Input: part model. Units: mm. Frame: model coordinates. A direction names the side the tool comes from. Coordinates: 2 decimals unless noted, no trailing zeros. Order: outer loops, then holes, each group sorted by start corner. A loop starts at its lowest first (then second) coordinate and runs counter-clockwise, first axis right, second up. Notation, with made-up numbers: M 37.5,1 L 85.5,1 A10 cw 85.5,6 Z; hole C 17,87 d1. An arc over 180 degrees is marked long. Answer in a Markdown table with one row per item.
from build123d import *

# Parameters (mm, degrees)
SKETCH1_R           = 4.198469776
BOSS_EXTRUDE1_DEPTH = 2


with BuildPart() as part:
    # Sketch1 → Boss-Extrude1 (new body)
    with BuildSketch(Plane(origin=(0, 0, 1287.795194646), x_dir=(-1, 0, 0), z_dir=(0, 0, -1))):
        with BuildLine():
            Line((-628.291713491, 871.098927157), (-628.291713491, 890.298927157))
            ThreePointArc((-628.291713491, 890.298927157), (-630.049072803, 894.541567844), (-634.291713491, 896.298927157))
            Line((-634.291713491, 896.298927157), (-714.691713491, 896.298927157))
            ThreePointArc((-714.691713491, 896.298927157), (-718.934354178, 894.541567844), (-720.691713491, 890.298927157))
            Line((-720.691713491, 890.298927157), (-720.691713491, 871.098927157))
            ThreePointArc((-720.691713491, 871.098927157), (-718.934354178, 866.85628647), (-714.691713491, 865.098927157))
            Line((-714.691713491, 865.098927157), (-634.291713491, 865.098927157))
            ThreePointArc((-634.291713491, 865.098927157), (-630.049072803, 866.85628647), (-628.291713491, 871.098927157))
        make_face()
        with Locations((-707.866713491, 880.098927157)):
            Circle(SKETCH1_R, mode=Mode.SUBTRACT)
        with Locations((-641.116713491, 880.098927157)):
            Circle(SKETCH1_R, mode=Mode.SUBTRACT)
        with BuildLine():
            Line((-682.991714253, 882.493927157), (-685.691713491, 882.493927157))
            Line((-685.691713491, 882.493927157), (-685.691713491, 891.298927157))
            Line((-685.691713491, 891.298927157), (-676.886713491, 891.298927157))
            Line((-676.886713491, 891.298927157), (-676.886713491, 888.59892792))
            ThreePointArc((-676.886713491, 888.59892792), (-677.027302174, 888.259516726), (-677.366713318, 888.11892792))
            Line((-677.366713318, 888.11892792), (-679.535834903, 888.118927139))
            ThreePointArc((-679.535834903, 888.118927139), (-680.090162448, 887.748537098), (-679.960098756, 887.09466307))
            Line((-679.960098756, 887.09466307), (-677.620321725, 884.754886039))
            ThreePointArc((-677.620321725, 884.754886039), (-676.705447884, 884.143586882), (-675.626280608, 883.928927162))
            Line((-675.626280608, 883.928927162), (-673.357146389, 883.928927157))
            ThreePointArc((-673.357146389, 883.928927157), (-672.277979107, 884.143586875), (-671.363105261, 884.754886034))
            Line((-671.363105261, 884.754886034), (-669.023328231, 887.094663064))
            ThreePointArc((-669.023328231, 887.094663064), (-668.893264539, 887.748537091), (-669.447592082, 888.118927133))
            Line((-669.447592082, 888.118927133), (-671.616713665, 888.11892792))
            ThreePointArc((-671.616713665, 888.11892792), (-671.956124807, 888.259516727), (-672.096713491, 888.59892792))
            Line((-672.096713491, 888.59892792), (-672.096713491, 891.298927157))
            Line((-672.096713491, 891.298927157), (-663.291713491, 891.298927157))
            Line((-663.291713491, 891.298927157), (-663.291713491, 882.493927157))
            Line((-663.291713491, 882.493927157), (-665.991712728, 882.493927157))
            ThreePointArc((-665.991712728, 882.493927157), (-666.331123921, 882.634515841), (-666.471712728, 882.973926984))
            Line((-666.471712728, 882.973926984), (-666.471713509, 885.14304857))
            ThreePointArc((-666.471713509, 885.14304857), (-666.84210355, 885.697376115), (-667.495977578, 885.567312423))
            Line((-667.495977578, 885.567312423), (-669.835754609, 883.227535392))
            ThreePointArc((-669.835754609, 883.227535392), (-670.447053766, 882.312661551), (-670.661713486, 881.233494275))
            Line((-670.661713486, 881.233494275), (-670.66171349, 878.964360056))
            ThreePointArc((-670.66171349, 878.964360056), (-670.447053773, 877.885192774), (-669.835754613, 876.970318927))
            Line((-669.835754613, 876.970318927), (-667.495977584, 874.630541898))
            ThreePointArc((-667.495977584, 874.630541898), (-666.842103556, 874.500478205), (-666.471713515, 875.054805749))
            Line((-666.471713515, 875.054805749), (-666.471712728, 877.223927331))
            ThreePointArc((-666.471712728, 877.223927331), (-666.331123921, 877.563338474), (-665.991712728, 877.703927157))
            Line((-665.991712728, 877.703927157), (-663.291713491, 877.703927157))
            Line((-663.291713491, 877.703927157), (-663.291713491, 868.898927157))
            Line((-663.291713491, 868.898927157), (-672.096713491, 868.898927157))
            Line((-672.096713491, 868.898927157), (-672.096713491, 871.598926394))
            ThreePointArc((-672.096713491, 871.598926394), (-671.956124807, 871.938337588), (-671.616713663, 872.078926394))
            Line((-671.616713663, 872.078926394), (-669.447592078, 872.078927176))
            ThreePointArc((-669.447592078, 872.078927176), (-668.893264533, 872.449317216), (-669.023328225, 873.103191245))
            Line((-669.023328225, 873.103191245), (-671.363105256, 875.442968275))
            ThreePointArc((-671.363105256, 875.442968275), (-672.277979097, 876.054267433), (-673.357146373, 876.268927152))
            Line((-673.357146373, 876.268927152), (-675.626280592, 876.268927157))
            ThreePointArc((-675.626280592, 876.268927157), (-676.705447874, 876.05426744), (-677.62032172, 875.44296828))
            Line((-677.62032172, 875.44296828), (-679.96009875, 873.103191251))
            ThreePointArc((-679.96009875, 873.103191251), (-680.090162442, 872.449317223), (-679.535834899, 872.078927182))
            Line((-679.535834899, 872.078927182), (-677.366713316, 872.078926394))
            ThreePointArc((-677.366713316, 872.078926394), (-677.027302174, 871.938337588), (-676.886713491, 871.598926394))
            Line((-676.886713491, 871.598926394), (-676.886713491, 868.898927157))
            Line((-676.886713491, 868.898927157), (-685.691713491, 868.898927157))
            Line((-685.691713491, 868.898927157), (-685.691713491, 877.703927157))
            Line((-685.691713491, 877.703927157), (-682.991714253, 877.703927157))
            ThreePointArc((-682.991714253, 877.703927157), (-682.65230306, 877.563338473), (-682.511714253, 877.22392733))
            Line((-682.511714253, 877.22392733), (-682.511713472, 875.054805744))
            ThreePointArc((-682.511713472, 875.054805744), (-682.141323432, 874.5004782), (-681.487449403, 874.630541892))
            Line((-681.487449403, 874.630541892), (-679.147672372, 876.970318923))
            ThreePointArc((-679.147672372, 876.970318923), (-678.536373215, 877.885192764), (-678.321713495, 878.96436004))
            Line((-678.321713495, 878.96436004), (-678.321713491, 881.233494258))
            ThreePointArc((-678.321713491, 881.233494258), (-678.536373208, 882.312661541), (-679.147672368, 883.227535387))
            Line((-679.147672368, 883.227535387), (-681.487449397, 885.567312417))
            ThreePointArc((-681.487449397, 885.567312417), (-682.141323425, 885.697376109), (-682.511713466, 885.143048566))
            Line((-682.511713466, 885.143048566), (-682.511714253, 882.973926983))
            ThreePointArc((-682.511714253, 882.973926983), (-682.65230306, 882.634515841), (-682.991714253, 882.493927157))
        make_face(mode=Mode.SUBTRACT)
    extrude(amount=BOSS_EXTRUDE1_DEPTH)


solid = part.part
1) Mould query, pull axis X, two halves, no side actions, for faces 1 (the face through (670.44, 882.33, 1286.81)), 2 (the face through (671, 888.119, 1287)), 3 (the face through (718.887, 894.588, 1286.809)), 4 (the face through (630, 894.49, 1286.81)). Classes: +X half, -X half, draft (parallel to the pull), parting line (faces both ways), or undercut.
Resolved:
| item | result |
|---|---|
| face 1 | undercut |
| face 2 | undercut |
| face 3 | +X half |
| face 4 | -X half |
2) Cut plane A-A, the plane x = 641.5. Output: boundary loops of the cut face in (y, z), and give its area (3 significant figures).
Resolved:
| item | result |
|---|---|
| outline | M 865.1,1285.8 L 875.92,1285.8 L 875.92,1287.8 L 865.1,1287.8 Z; M 884.28,1285.8 L 896.3,1285.8 L 896.3,1287.8 L 884.28,1287.8 Z |
| area | 45.7 mm2 |
3) Reachability of faces 5 (the face through (676.887, 890, 1287)), 6 (the face through (675.1, 884.4, 1285.795)) from +Z, -Z, +X, -X, +Y, -Y: full face, straight path, thin tool, end or side. Return the list, or none.
Resolved:
| item | result |
|---|---|
| face 5 | +Z, -Z |
| face 6 | -Z, +X, -X, +Y, -Y |
4) Material intervals for probe 1 along Y at (x, z) = (684.5, 1287.35); probe 2 along Y at (x, z) = (674, 1287.1); probe 3 along X at (y, z) = (881, 1286.5), sorted ascending.
Resolved:
| item | result |
|---|---|
| probe 1 | y = 865.1 to 868.9, 877.7 to 882.49, 891.3 to 896.3 |
| probe 2 | y = 865.1 to 876.27, 883.93 to 896.3 |
| probe 3 | x = 628.29 to 637.02, 645.22 to 670.66, 678.32 to 703.77, 711.97 to 720.69 |
5) Cut plane B-B, the plane z = 1286.4. State how many separate pieces and enclosed holes the cut face has, and give its area (3 significant figures).
Resolved:
| item | result |
|---|---|
| separate pieces | 1 |
| enclosed holes | 3 |
| area | 2,440 mm2 |
6) Contact query for a flat-ended pin moving along its axis: pin 1 (8 mm diameter, centred on x = 644, y = 880, fed in from +Z). Output: stop coordinate, or through.
Resolved:
| item | result |
|---|---|
| pin 1 | stops at z = 1287.8 |
